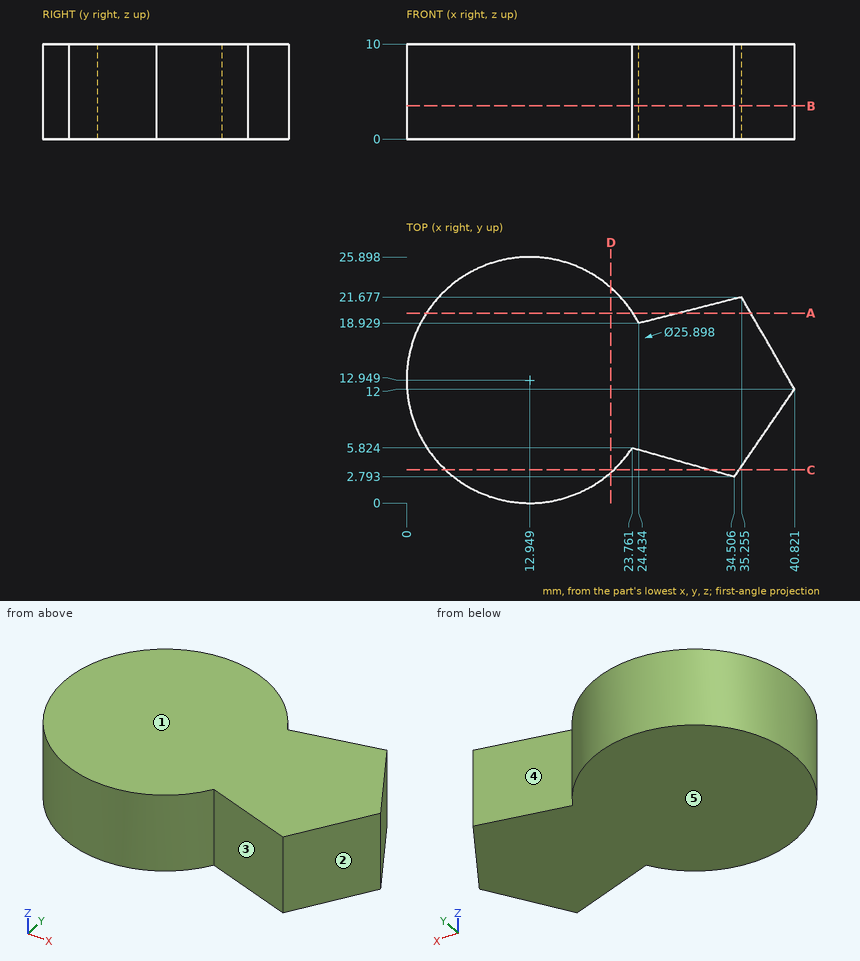
Input: dimensioned drawing with shaded views. Units: mm. Origin: part minimum x, y, z. A direction names the side the tool comes from. Give positions to 0.01 mm unless a question says otherwise; leave off trailing zeros. Order: outer loops, then holes, each group sorted by start corner. A loop starts at its lowest first (then second) coordinate and runs counter-clockwise, first axis right, second up.
(1) Pull-direction query (X, two-part tool) for the marked faces 1, 2 and 3; classes: +X half, -X half, draft (parallel to the pull), parting line (faces both ways), or undercut.
(2) Material intervals for line 1 along Y through (x, z) = (36, 1.5) (1 decimal); line 2 along Y through (x, z) = (14.5, 5.5) (1 decimal); line 3 along X through (y, z) = (8, 8) (1 decimal), sorted ascending.
(3) Access query for the marked faces 4 and 5. Directions: +Z, -Z, +X, -X, +Y, -Y. A direction counts if a zero-diameter tool reaches every point of the face in a straight line with its end or side. Return the directions, or none.
(4) Section query D-D (x = 21.5). Return the cut outline in (y, z) (1 decimal).
(5) Section query C-C (y = 3.5). Return the cut outline in (x, z) (1 decimal).
(6) Section query A-A (y = 20). Return the cut outline in (x, z).
(7) Section query B-B (z = 3.5). Return the cut outline in (x, y) (1 decimal), plus the area to 3 significant figures.
(8) Contact query for flat-ended pins moving along their axis: P1, Ø2, axis at x = 33, z = 3.5, coming from the +Y side; P2, Ø2, axis at x = 27.5, z = 3, coming from the -Y side; P3, Ø1.5, axis at x = 11.5, z = 1.5, coming from the -Y side. Output: stop coordinate, or through.
Outcome:
1. face 1: draft
1. face 2: +X half
1. face 3: undercut
2. line 1: y = 5 to 20.4
2. line 2: y = 0.1 to 25.8
2. line 3: x = 1 to 38.1
3. face 4: +Z, -Z, +Y
3. face 5: -Z, +X, -X, +Y, -Y
4. outline: (3.2, 0) - (22.7, 0) - (22.7, 10) - (3.2, 10) - close
5. outline: (4.1, 0) - (21.8, 0) - (21.8, 10) - (4.1, 10) - close; (32, 0) - (35, 0) - (35, 10) - (32, 10) - close
6. outline: (2.09, 0) - (23.81, 0) - (23.81, 10) - (2.09, 10) - close; (28.65, 0) - (36.22, 0) - (36.22, 10) - (28.65, 10) - close
7. outline: (23.8, 5.8) - (34.5, 2.8) - (40.8, 12) - (35.3, 21.7) - (24.4, 18.9) arc R12.9 ccw (long way) to start
7. area: 740 mm2
8. P1: stops at y = 21.36
8. P2: stops at y = 4.49
8. P3: stops at y = 0.02
